Answer from the drawing. Dimensions are ordinates in mm from the lowest x, y and z of the part. A direction names the side the tool comes from. Give positions to 0.01 mm unless a question says otherwise; leave off trailing zeros. Loops run counter-clockwise (first coordinate to the right, second up) from the corner with the lowest first, then second, coordinate; pieces in that order, holes last. Notation, with made-up numbers: (-14.5, 81.25) - (-5.5, 81.25) arc R9 cw to (-5.5, 92.25) - close; hole circle Ø9 at (61.25, 38). An arc over 180 degrees is marked (long way). One line per item, written item: value.
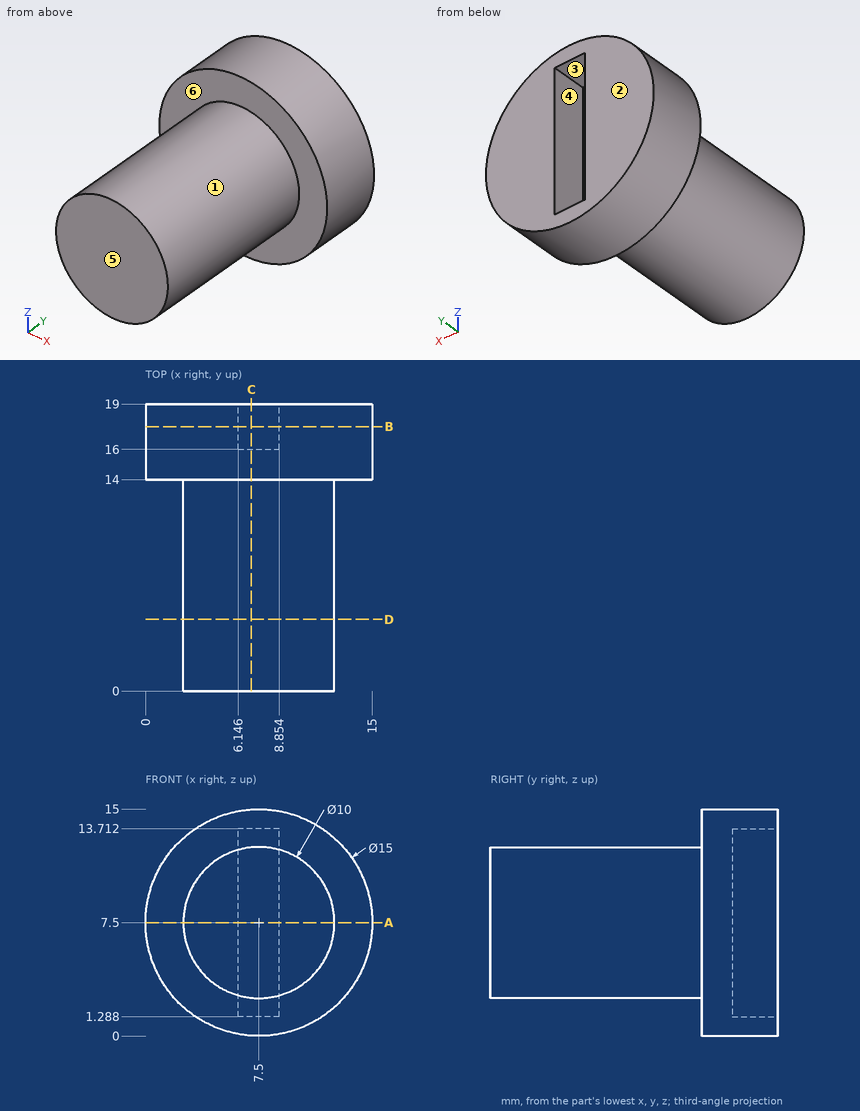
1. Flat-ended cylindrical pins translate along their axes: pin 1 Ø1.5 at (y, z) = (17, 5.5) entering from -X (1 decimal); pin 2 Ø8 at (y, z) = (4.5, 9.5) entering from -X; pin 3 Ø1.5 at (y, z) = (2.5, 10.5) entering from -X (1 decimal). Find the tip coordinate at first contact, or state that the pin passes through.
Output:
pin 1: stops at x = 0.1
pin 2: stops at x = 2.5
pin 3: stops at x = 3
2. For the marked faces 5 and 6, determine the directions among +Z, -Z, +X, -X, +Y, -Y from which every point of the face is accessible in a straight line to the end or side of a thin tool.
Output:
face 5: +Z, -Z, +X, -X, -Y
face 6: -Y
3. The mould has two halves that part along Z. Classify the marked faces 1, 2, 3 and 4: released by +Z, released by -Z, zero draft, split by the parting line, or undercut.
Output:
face 1: split by the parting line
face 2: zero draft
face 3: undercut
face 4: undercut
4. Section B-B (y = 17.5) is taken. Write down the section's boundary in (x, z).
Output:
outline: circle Ø15 at (7.5, 7.5); hole (6.15, 1.29) - (8.85, 1.29) - (8.85, 13.71) - (6.15, 13.71) - close
5. Section C-C (x = 7) is taken. Write down the section's boundary in (y, z) (1 decimal), and give its area (3 significant figures).
Output:
outline: (0, 2.5) - (14, 2.5) - (14, 0) - (19, 0) - (19, 1.3) - (16, 1.3) - (16, 13.7) - (19, 13.7) - (19, 15) - (14, 15) - (14, 12.5) - (0, 12.5) - close
area: 177 mm²
6. Section D-D (y = 4.75) is taken. Write down the section's boundary in (x, z).
Output:
outline: circle Ø10 at (7.5, 7.5)
7. Find the intervals of material crossed by line 1 along Y through (x, z) = (13, 7.5); line 2 along X through (y, z) = (16.25, 12.75) (1 decimal); line 3 along Y through (x, z) = (7.25, 2), in increasing order.
Output:
line 1: y = 14 to 19
line 2: x = 2.1 to 6.1, 8.9 to 12.9
line 3: y = 14 to 16
8. Section A-A (z = 7.5) is taken. Write down the section's boundary in (x, y).
Output:
outline: (0, 14) - (2.5, 14) - (2.5, 0) - (12.5, 0) - (12.5, 14) - (15, 14) - (15, 19) - (8.85, 19) - (8.85, 16) - (6.15, 16) - (6.15, 19) - (0, 19) - close
